Build history of the part. All positions in model axes, mm. Coordinates: 2 decimals unless noted, no trailing zeros. Loops run counter-clockwise (first coordinate to the right, second up) from the corner with the lowest first, then second, coordinate; pieces in that order, holes last. Notation, with made-up numbers: (-34.5, 66) - (15.5, 66) arc R26 ccw to (15.5, 101) - close; hole circle Ø6 at (-31.75, -34). An arc over 180 degrees is marked (long way). One line per item, written item: value.
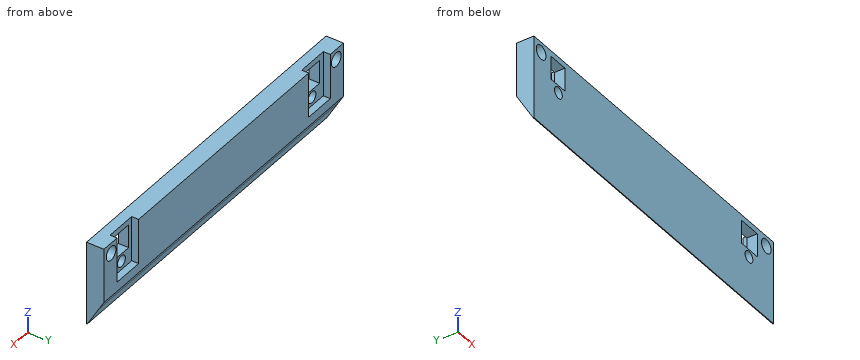
```python
from build123d import *

# Parameters (mm, degrees)
CROQUIS1_W                 = 100
CROQUIS1_H                 = 24
CROQUIS1_R                 = 2.017504942
CROQUIS1_W_2               = 5.897168216
CROQUIS1_H_2               = 6.754663932
CROQUIS1_W_3               = 6.477766384
SALIENTE_EXTRUIR1_DEPTH    = 5
CROQUIS2_W                 = 9
CROQUIS2_H                 = 13
CROQUIS2_R                 = 2.5
CORTAR_EXTRUIR1_DEPTH      = 2
CORTAR_EXTRUIR5_DEPTH      = 141
CORTAR_EXTRUIR6_DEPTH      = 21
CORTAR_EXTRUIR6_DEPTH_BACK = 26
CROQUIS5_R                 = 1.626798587


with BuildPart() as part:
    # Croquis1 → Saliente-Extruir1 (new body)
    with BuildSketch(Plane(origin=(0, 0, 0), x_dir=(1, 0, 0), z_dir=(0, 1, 0))):
        Rectangle(CROQUIS1_W, CROQUIS1_H)
        with Locations(Location((-47, -9, 0), (0, 0, 270))):
            Circle(CROQUIS1_R, mode=Mode.SUBTRACT)
        with Locations(Location((47, -9, 0), (0, 0, 270))):
            Circle(CROQUIS1_R, mode=Mode.SUBTRACT)
        with Locations((-40, -7)):
            Rectangle(CROQUIS1_W_2, CROQUIS1_H_2, mode=Mode.SUBTRACT)
        with Locations((40, -7)):
            Rectangle(CROQUIS1_W_3, CROQUIS1_H_2, mode=Mode.SUBTRACT)
    extrude(amount=SALIENTE_EXTRUIR1_DEPTH)

    # Croquis2 → Cortar-Extruir1 (cut)
    # profile 1 of 2: a face of its own
    with BuildSketch(Plane(origin=(0, 5, 0), x_dir=(1, 0, 0), z_dir=(0, 1, 0))):
        with Locations((-40, -5.5)):
            Rectangle(CROQUIS2_W, CROQUIS2_H)
        with Locations((-40, -7)):
            Circle(CROQUIS2_R, mode=Mode.SUBTRACT)
    # profile 2 of 2: a face of its own
    with BuildSketch(Plane(origin=(0, 5, 0), x_dir=(1, 0, 0), z_dir=(0, 1, 0))):
        with Locations((40, -5.5)):
            Rectangle(CROQUIS2_W, CROQUIS2_H)
        with Locations((40, -7)):
            Circle(CROQUIS2_R, mode=Mode.SUBTRACT)
    extrude(amount=-CORTAR_EXTRUIR1_DEPTH, mode=Mode.SUBTRACT)

    # Croquis3 → Cortar-Extruir5 (cut)
    with BuildSketch(Plane.ZY.offset(50)):
        Polygon((-12, 5), (-12, 0.2), (-6.100895765, 3.605849418), (-3.686156124, 5), align=None)
        Polygon((-12.757171087, 0.2), (-12, 0.2), (-12, 5), (-3.686156124, 5), (-3.039853353, 5.373143079), (-12.757171087, 5.373143079), align=None)
    extrude(amount=-CORTAR_EXTRUIR5_DEPTH, mode=Mode.SUBTRACT)

    # Croquis5 → Cortar-Extruir6 (cut, two sides: drawn at the far end of the back side and taken through both)
    with BuildSketch(Plane(origin=(0, 3, 0), x_dir=(1, 0, 0), z_dir=(0, 1, 0)).offset(-CORTAR_EXTRUIR6_DEPTH_BACK)):
        with Locations(Location((39.778371373, -1.459300721, 0), (0, 0, 270))):
            Circle(CROQUIS5_R)
        with Locations(Location((-39.778371373, -1.459300721, 0), (0, 0, 270))):
            Circle(CROQUIS5_R)
    extrude(amount=CORTAR_EXTRUIR6_DEPTH + CORTAR_EXTRUIR6_DEPTH_BACK, mode=Mode.SUBTRACT)


solid = part.part
```
Item 1: Probe probe 1 along X at (y, z) = (4.35, 5.75); probe 2 along X at (y, z) = (2.8, 9); probe 3 along X at (y, z) = (4.5, 9). List the from-to ranges inside material, lowest first. Write a range as from..to.
Check result:
probe 1: x = -50..-44.5, -35.5..35.5, 44.5..50
probe 2: x = -50..-49.02, -44.98..-42.95, -37.05..36.76, 43.24..44.98, 49.02..50
probe 3: x = -50..-49.02, -44.98..-44.5, -35.5..35.5, 44.5..44.98, 49.02..50
Item 2: Cut at D-D, the plane y = 1.15. Write the cut outline in (x, z) (1 decimal).
Check result:
outline: (-50, -10.4) - (50, -10.4) - (50, 12) - (-50, 12) - close; hole circle Ø4 at (-47, 9); hole (-42.9, 3.6) - (-37.1, 3.6) - (-37.1, 10.4) - (-42.9, 10.4) - close; hole circle Ø3.3 at (-39.8, 1.5); hole (36.8, 3.6) - (43.2, 3.6) - (43.2, 10.4) - (36.8, 10.4) - close; hole circle Ø3.3 at (39.8, 1.5); hole circle Ø4 at (47, 9)
Item 3: Cut at B-B, the plane z = 9. Write the cut outline in (x, y), then the cut area to 3 significant figures.
Check result:
outline: (-50, 0) - (-49.02, 0) - (-49.02, 5) - (-50, 5) - close; (-44.98, 0) - (-42.95, 0) - (-42.95, 3) - (-44.5, 3) - (-44.5, 5) - (-44.98, 5) - close; (-37.05, 0) - (36.76, 0) - (36.76, 3) - (35.5, 3) - (35.5, 5) - (-35.5, 5) - (-35.5, 3) - (-37.05, 3) - close; (43.24, 0) - (44.98, 0) - (44.98, 5) - (44.5, 5) - (44.5, 3) - (43.24, 3) - close; (49.02, 0) - (50, 0) - (50, 5) - (49.02, 5) - close
area: 387 mm^2
Item 4: Drop flat-ended pins along their axis: P1, Ø3.5, axis at x = 39.78, z = 1.46, coming from the +Y side; P2, Ø2.5, axis at x = -47, z = 9, coming from the +Y side; P3, Ø1, axis at x = 39.5, y = 4, coming from the +Z side. Give the stop position or say it passes through.
Check result:
P1: stops at y = 3
P2: passes through
P3: stops at z = -1
Item 5: Cut at C-C, the plane z = 1.25. Write the cut outline in (x, y), then the cut area to 3 significant figures.
Check result:
outline: (-50, 0) - (-41.39, 0) - (-41.39, 3) - (-44.5, 3) - (-44.5, 5) - (-50, 5) - close; (-38.17, 0) - (38.17, 0) - (38.17, 3) - (35.5, 3) - (35.5, 5) - (-35.5, 5) - (-35.5, 3) - (-38.17, 3) - close; (41.39, 0) - (50, 0) - (50, 5) - (44.5, 5) - (44.5, 3) - (41.39, 3) - close
area: 445 mm^2
Item 6: Cut at A-A, the plane x = 47. Write the cut outline in (y, z), then the cut area to 3 significant figures.
Check result:
outline: (0, -12) - (0.2, -12) - (5, -3.69) - (5, 6.98) - (0, 6.98) - close; (0, 11.02) - (5, 11.02) - (5, 12) - (0, 12) - close
area: 79.9 mm^2
